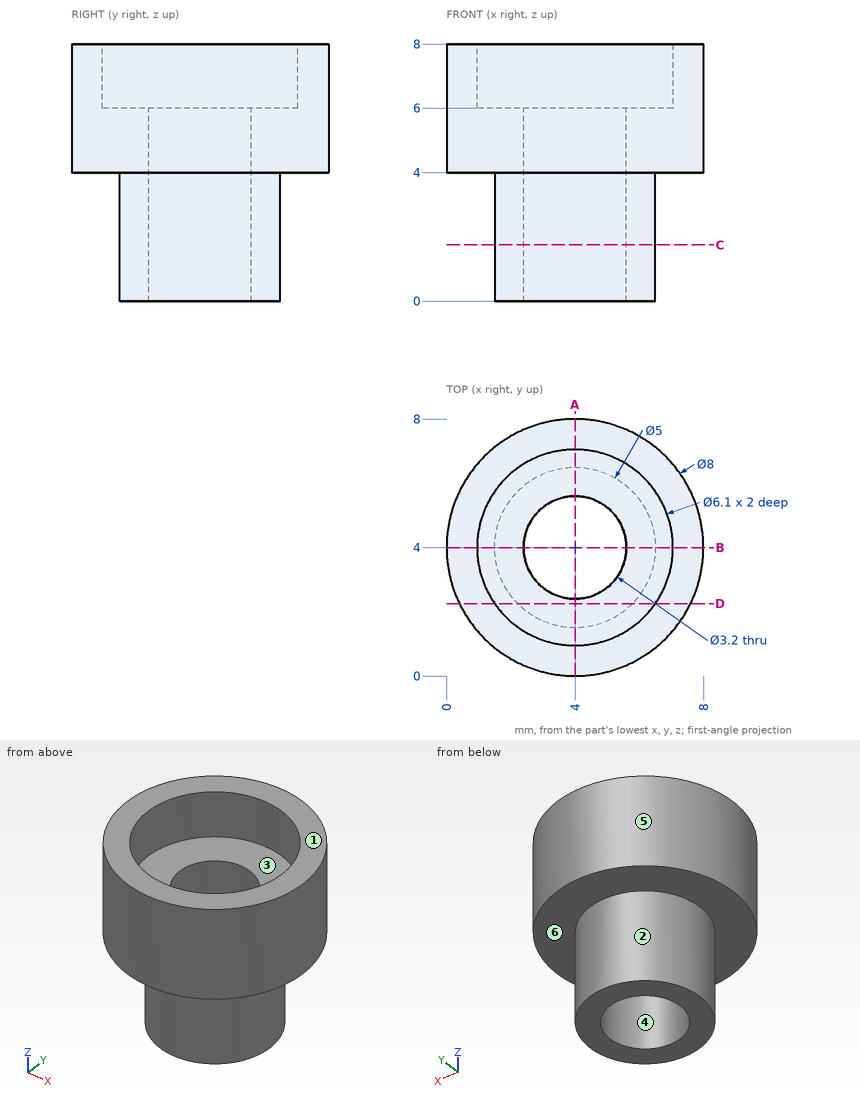
Input: dimensioned drawing with shaded views. Units: mm. Origin: part minimum x, y, z. A direction names the side the tool comes from. Give positions to 0.01 mm unless a question says otherwise; leave off trailing zeros. Loops run counter-clockwise (first coordinate to the right, second up) from the corner with the lowest first, then second, coordinate; pieces in that order, holes last. Notation, with made-up numbers: M -29.75,71.5 L -15.75,71.5 A19 ccw -15.75,87.5 Z; hole C -20,-29 d7. An arc over 180 degrees is marked long. Put each result on its own line as item: value. Start each with the question number.
1) Pull-direction query (Y, two-part tool) for the marked faces 4, 5 and 6; classes: pulls with the +Y half, pulls with the -Y half, needs draft (parallel to the pull), parting line crosses it, or undercut.
2) Cut plane A-A (x = 4). Output: boundary loops of the cut face in (y, z), then the cut area to 3 significant figures.
3) Access query for the marked faces 1, 2 and 3. Directions: +Z, -Z, +X, -X, +Y, -Y. A direction counts if a zero-diameter tool reaches every point of the face in a straight line with its end or side. Return the directions, or none.
4) Cut plane D-D (y = 2.25). Output: boundary loops of the cut face in (x, z), then the cut area to 3 significant figures.
5) Contact query for flat-ended pins moving along their axis: pin 1 (4 mm diameter, centred on x = 4.5, y = 3.5, fed in from -Z); pin 2 (3.5 mm diameter, centred on x = 4, y = 4, fed in from +Z); pin 3 (1 mm diameter, centred on x = 2.5, z = 5, fed in from +Y). Output: stop coordinate, or through.
6) Cut plane C-C (z = 1.75). Output: boundary loops of the cut face in (x, y).
7) Ray query, line 1 along Y through (x, z) = (4, 7); line 2 along X through (y, z) = (4.75, 4.25); line 3 along X through (y, z) = (4.25, 6.75). Return the intervals inside material, ascending.
Verdict:
1. face 4: undercut
1. face 5: parting line crosses it
1. face 6: needs draft
2. outline: M 0,4 L 1.5,4 L 1.5,0 L 2.4,0 L 2.4,6 L 0.95,6 L 0.95,8 L 0,8 Z; M 5.6,0 L 6.5,0 L 6.5,4 L 8,4 L 8,8 L 7.05,8 L 7.05,6 L 5.6,6 Z
2. area: 20.6 mm2
3. face 1: +Z, +X, -X, +Y, -Y
3. face 2: -Z
3. face 3: +Z
4. outline: M 0.4,4 L 2.21,4 L 2.21,0 L 5.79,0 L 5.79,4 L 7.6,4 L 7.6,8 L 6.5,8 L 6.5,6 L 1.5,6 L 1.5,8 L 0.4,8 Z
4. area: 33.1 mm2
5. pin 1: z = 0
5. pin 2: z = 6
5. pin 3: y = 7.87
6. outline: C 4,4 d5; hole C 4,4 d3.2
7. line 1: 0 to 0.95, 7.05 to 8
7. line 2: 0.07 to 2.59, 5.41 to 7.93
7. line 3: 0.01 to 0.96, 7.04 to 7.99
